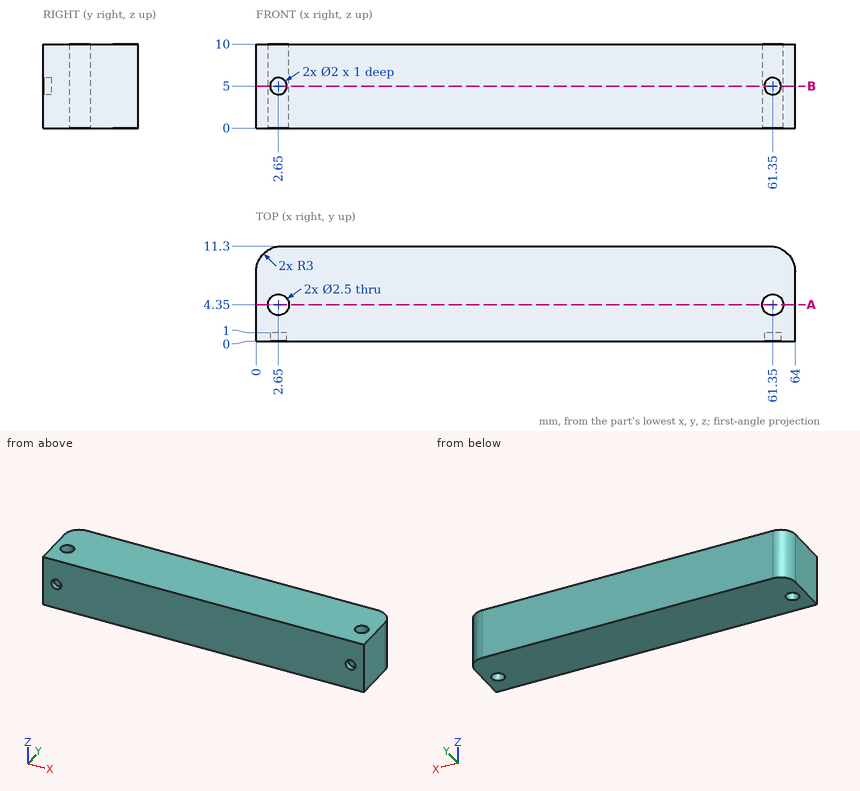
Can you work these out from the drawing? Everything is in mm from the part's minimum corner. Round coordinates to 2 decimals unless told otherwise and drop trailing zeros. Loops run counter-clockwise (first coordinate to the right, second up) from the corner with the lowest first, then second, coordinate; pieces in that order, holes last. Notation, with made-up numbers: (0.5, 87) - (52.5, 87) arc R26 cw to (52.5, 122) - close; hole circle Ø3 at (63, 61). An arc over 180 degrees is marked (long way). Answer as CSV lines item,"result".
1. For pin 1 Ø2 at (x, y) = (2.65, 4.35) entering from -Z, with a flat end and sliding along its axis, tell me the tip position at first contact or that it passes through.
Filled in:
pin 1,"passes through"
2. I want a section at B-B on z = 5. List the corners of the cut face in (x, y) for me.
Filled in:
outline,"(0, 0) - (1.65, 0) - (1.65, 1) - (3.65, 1) - (3.65, 0) - (60.35, 0) - (60.35, 1) - (62.35, 1) - (62.35, 0) - (64, 0) - (64, 8.3) arc R3 ccw to (61, 11.3) - (3, 11.3) arc R3 ccw to (0, 8.3) - close; hole circle Ø2.5 at (2.65, 4.35); hole circle Ø2.5 at (61.35, 4.35)"
3. Please list where these lines run through material, in increasing order: line 1 along X through (y, z) = (4.35, 4); line 2 along Z through (x, y) = (2.65, 0.4); line 3 along Y through (x, z) = (2.65, 4.5). Write a range as [from, to].
Filled in:
line 1,"x = [0, 1.4], [3.9, 60.1], [62.6, 64]"
line 2,"z = [0, 4], [6, 10]"
line 3,"y = [1, 3.1], [5.6, 11.28]"
4. I want a section at A-A on y = 4.35. List the corners of the cut face in (x, z) for me, then the cut area to 3 significant figures.
Filled in:
outline,"(0, 0) - (1.4, 0) - (1.4, 10) - (0, 10) - close; (3.9, 0) - (60.1, 0) - (60.1, 10) - (3.9, 10) - close; (62.6, 0) - (64, 0) - (64, 10) - (62.6, 10) - close"
area,"590 mm^2"
